Check sheet for the modelled part. Datum: model origin and axes. Units: mm. A direction names the side the tool comes from. Give positions to 0.01 mm unless a question says otherwise; leave off trailing zeros. Write each loop counter-clockwise with the first axis right and the second up, starting at its lowest first coordinate (ties: lowest second). Pieces come first, ordered by that corner, then holes. Notation, with made-up numbers: (29, -28) -> (47, -28) arc R25 cw to (47, -4) -> close; hole circle Ø2 at (10.25, 80). An arc over 180 degrees is marked (long way). Use a Markdown table: item, result. Add a question column.
1. Cross-section at C-C (z = -17). Enter the section's corners in (x, y).
2. Cross-section at D-D (x = 9.5). Enter the section's corners in (y, z), then the cut area to 3 significant figures.
3. Cross-section at B-B (x = 0). Enter the section's corners in (y, z).
4. Scan lines: probe 1 along X at (y, z) = (-0.25, -13); probe 2 along Z at (x, y) = (-8.75, -2.75); probe 3 along Z at (x, y) = (-6.25, -10.25). Record each from-to range of solid material in increasing order. Write a range as [from, to].
5. Set-up check for faces 1 (the flat face through (-3, -5.4, -10)), 2 (the cylindrical face through (5.77, 11.09, -5.07)), 3 (the flat face through (0, -9, -5)): record each of +Z, -Z, +X, -X, +Y, -Y from which the full face is reachable in a straight line by a thin tool's end or side.
6. Gauge pin test, flat ends, axial feed: P1, Ø8, axis at x = 9, z = -12.5, coming from the -Y side; P2, Ø4, axis at y = 1, z = -21, coming from the -X side; P3, Ø12, axis at x = -7.5, y = 0.5, coming from the +Z side; P4, Ø3, axis at y = -4, z = -26.5, coming from the -X side. Record the tip position at first contact, or that the pin passes through.
7. Cross-section at A-A (y = 0). Enter the section's corners in (x, z), then the cut area to 3 significant figures.
Solid Edge part; units mm, degrees
sketch "Sketch1" plane through (0, 0, 0) normal (0, -1, 0) x (1, 0, 0)
  line L0 (0, 0) -> (12.5, 0)
  line L1 (12.5, 0) -> (12.5, -10)
  line L2 (12.5, -10) -> (6, -10)
  line L3 (6, -10) -> (6, -40)
  line L4 (6, -40) -> (0, -40)
  dimension "D1" = 12.5
revolve "RevolvedProtrusion1" add sketch "Sketch1" angle 360 about axis through (0, 0, -20) along (0, 0, 1)
sketch "Sketch2" plane through (0, 0, 0) normal (0, 0, 1) x (1, 0, 0)
  line L0 (-10.3562, -7) -> (10.3562, -7)
extrude "Cutout1" cut sketch "Sketch2" against normal blind 5 material side at (0, -7.05, 0)
Worked answers:
| question | item | result |
|---|---|---|
| 1 | outline | circle Ø12 at (0, 0) |
| 2 | outline | (-8.12, -10) -> (8.12, -10) -> (8.12, 0) -> (-7, 0) -> (-7, -5) -> (-8.12, -5) -> close |
| 2 | area | 157 mm² |
| 3 | outline | (-12.5, -10) -> (-6, -10) -> (-6, -40) -> (6, -40) -> (6, -10) -> (12.5, -10) -> (12.5, 0) -> (-7, 0) -> (-7, -5) -> (-12.5, -5) -> close |
| 4 | probe 1 | x = [-5.99, 5.99] |
| 4 | probe 2 | z = [-10, 0] |
| 4 | probe 3 | z = [-10, -5] |
| 5 | face 1 | -Z |
| 5 | face 2 | +Z, -Z |
| 5 | face 3 | +Z, +X, -X, -Y |
| 6 | P1 | stops at y = -11.03 |
| 6 | P2 | stops at x = -6 |
| 6 | P3 | stops at z = 0 |
| 6 | P4 | stops at x = -5.45 |
| 7 | outline | (-12.5, -10) -> (-6, -10) -> (-6, -40) -> (6, -40) -> (6, -10) -> (12.5, -10) -> (12.5, 0) -> (-12.5, 0) -> close |
| 7 | area | 610 mm² |
